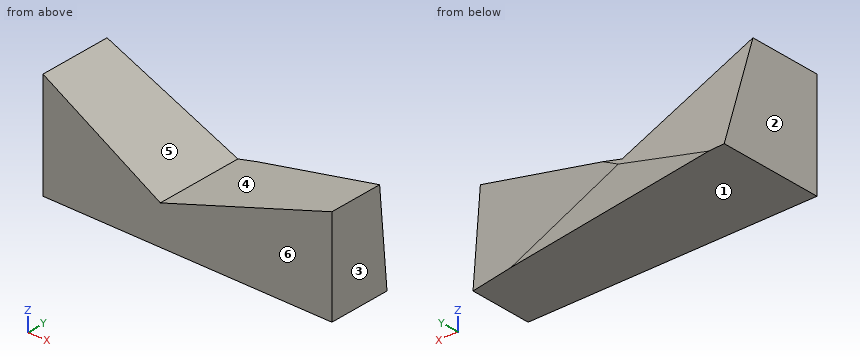
Autodesk Inventor part; units mm, degrees
ref_plane "YZ Plane" through (0, 0, 0) normal (1, 0, 0) x (0, 1, 0)
ref_plane "XZ Plane" through (0, 0, 0) normal (0, 1, 0) x (-1, 0, 0)
ref_plane "XY Plane" through (0, 0, 0) normal (0, 0, 1) x (1, 0, 0)
sketch "スケッチ5" plane through (0, 0, 0) normal (0, 1, 0) x (-1, 0, 0)
  line L0 (-559.0798, 16.0883) -> (-559.0798, -283.3342)
  line L1 (-559.0798, -283.3342) -> (344.6263, -283.3342)
  line L2 (344.6263, -283.3342) -> (344.6263, 47.8084)
  line L3 (-559.0798, 16.0883) -> (-22.4967, -162.5803)
  line L4 (-22.4967, -162.5803) -> (344.6263, 47.8084)
  point P0 (0, 0)
extrude "押し出し5" add sketch "スケッチ5" along normal blind 360
sketch3d "3D スケッチ1"
ref_plane "作業平面1" through (557.1342, 171.5665, 5.3514) normal (0.1727, 0.9812, 0.0862) x (-0.2514, 0.1285, -0.9593)
ref_plane "作業平面4" through (-344.5976, 233.5337, 31.5954) normal (-0.0442, -0.9544, -0.2952) x (-0.0031, 0.2956, -0.9553)
ref_plane "作業平面5" through (-345.6786, 336.3426, -300.6801) normal (0.1489, 0.9888, -0.0028) x (0.9391, -0.1406, 0.3137)
sketch "スケッチ6" plane through (557.1342, 171.5665, 5.3514) normal (0.1727, 0.9812, 0.0862) x (-0.2514, 0.1285, -0.9593)
  line L0 (-514.7241, -766.6326) -> (967.6123, -766.6326)
  line L1 (967.6123, -766.6326) -> (967.6123, 1684.2947)
  line L2 (967.6123, 1684.2947) -> (-514.7241, 1684.2947)
  line L3 (-514.7241, 1684.2947) -> (-514.7241, -766.6326)
  point P0 (123.1359, 504.4343)
sketch "スケッチ7" plane through (-345.6786, 336.3426, -300.6801) normal (0.1489, 0.9888, -0.0028) x (0.9391, -0.1406, 0.3137)
  line L0 (2221.5026, -667.2238) -> (-1676.0607, -667.2238)
  line L1 (-1676.0607, -667.2238) -> (-1676.0607, 746.6169)
  line L2 (-1676.0607, 746.6169) -> (2221.5026, 746.6169)
  line L3 (2221.5026, 746.6169) -> (2221.5026, -667.2238)
  point P0 (466.2154, -161.8023)
sketch "スケッチ8" plane through (-344.5976, 233.5337, 31.5954) normal (-0.0442, -0.9544, -0.2952) x (-0.0031, 0.2956, -0.9553)
  line L0 (-1292.5456, 2575.2008) -> (1231.0674, 2575.2008)
  line L1 (1231.0674, 2575.2008) -> (1231.0674, -1866.358)
  line L2 (1231.0674, -1866.358) -> (-1292.5456, -1866.358)
  line L3 (-1292.5456, -1866.358) -> (-1292.5456, 2575.2008)
  point P0 (-39.9159, 354.4214)
extrude "押し出し6" cut sketch "スケッチ7" along normal blind 360
extrude "押し出し7" cut sketch "スケッチ8" against normal blind 360
extrude "押し出し8" cut sketch "スケッチ6" along normal blind 360
properties part number "wall"
The listing builds one solid part. Answer for the finished solid, in the listing's coordinates (mm). Face numbers are marked on the shaded views. A direction names the side the tool comes from. Give positions to 0.01 mm unless a question says otherwise; leave off trailing zeros. Order: outer loops, then holes, each group sorted by start corner. A loop starts at its lowest first (then second) coordinate and runs counter-clockwise, first axis right, second up. Notation, with made-up numbers: M 78,-4 L 118,-4 A34 ccw 118,32 Z; hole C -30.75,83 d9. An arc over 180 degrees is marked long. Put each result on its own line as item: value. Start each with the question number.
Item 1: Which of the six approach directions +Z, -Z, +X, -X, +Y, -Y give full straight-line access (tool end or side, diameter ignored) to the marked faces 5 and 6?
Item 2: The part is cut by section D-D, the plane z = 6.5. Determine the outline of the cut face in (x, y).
Item 3: The part is cut by section B-B, the plane y = 121.5. Determine the outline of the cut face in (x, z), and give its area (3 significant figures).
Item 4: The part is cut by section A-A, the plane z = -124. Determine the outline of the cut face in (x, y), and give its area (3 significant figures).
Item 5: Flat-ended cylindrical pins translate along their axes: P1, Ø1.5, axis at x = -76, z = -190.5, coming from the +Y side; P2, Ø4, axis at x = 218.5, y = 56, coming from the +Z side; P3, Ø4, axis at x = 117, y = 207, coming from the +Z side. Find the tip coordinate at first contact, or state that the pin passes through.
Item 6: Find the intervals of material crossed by line 1 along Z through (x, y) = (-4.5, 65); line 2 along Y through (x, z) = (387.5, -190); line 3 along Y through (x, z) = (350, -175), in increasing order.
Item 7: The part is cut by section C-C, the plane x = 45.5. Determine the outline of the cut face in (y, z).
Item 8: For a pull along X with two mould halves and no side action, classify the marked faces 1, 2, 3 and 4 as +X half, -X half, draft (parallel to the pull), parting line (faces both ways), or undercut.
Answer key:
1. face 5: +Z, +Y, -Y
1. face 6: +Z, -Z, +X, -X, -Y
2. outline: M -344.63,0 L -272.54,0 L -272.54,237.96 L -344.63,241.3 Z; M 530.28,0 L 559.08,0 L 559.08,171.12 L 530.28,176.19 Z
3. outline: M -344.63,-283.33 L 559.08,-283.33 L 559.08,16.09 L 22.5,-162.58 L -344.63,47.81 Z
3. area: 196,000 mm²
4. outline: M -344.63,0 L -44.82,0 L -44.82,267.77 L -344.63,281.66 Z; M 138.36,0 L 559.08,0 L 559.08,182.59 L 138.36,256.64 Z
4. area: 175,000 mm²
5. P1: stops at y = 290.02
5. P2: stops at z = -96.65
5. P3: stops at z = -130.45
6. line 1: z = -283.33 to -147.11
6. line 2: y = 0 to 218.58
6. line 3: y = 0 to 223.87
7. outline: M 0,-283.33 L 277.48,-283.33 L 277.78,-178.63 L 276.7,-166.4 L 273.16,-154.92 L 0,-154.92 Z
8. face 1: draft
8. face 2: -X half
8. face 3: +X half
8. face 4: undercut
